Model file for the job. Use its own axes, mm. A direction names the side the tool comes from. Give positions to 0.01 mm unless a question says otherwise; leave off trailing zeros. Order: outer loops, then holes, each group sorted by start corner. A loop starts at its lowest first (then second) coordinate and runs counter-clockwise, first axis right, second up. Notation, with made-up numbers: M 65,76.25 L 113,76.25 A21 cw 113,103.25 Z; hole C 71,-5 d9. An arc over 180 degrees is marked long. Return JSON: item names as keys, results as strings. Group by question number.
1. Wall check: probe 1 along X at (y, z) = (0, -3.5); probe 2 along X at (y, z) = (1, -6). Give the ranges that are in metal, low to high. Write a range as [from, to].
2. Two-plate mould, pull along X, no slides. Class faces 4 (the face through (0, 1, 1)), 5 (the face through (2.11, -5.85, 1.34)), 6 (the face through (1, 0, 1)): released by +X, released by -X, zero draft, split by the parting line, or undercut.
3. 3-axis set-ups, long thin cutter, end or side, ignore diameter. For faces 1 (the face through (1.34, 2.11, -5.85)), 2 (the face through (1, 1, 0)), 3 (the face through (-5.85, 1.69, 1.84)): which of +Z, -Z, +X, -X, +Y, -Y reach the whole face in a straight line?
4. Slice it at D-D on x = -6.75. List the corners of the cut face in (y, z), then the cut area to 3 significant figures.
5. Pin check, flat tips, straight feed: pin 1 (10 mm diameter, centred on x = 5, y = -5.5, fed in from +Z); pin 2 (4.5 mm diameter, centred on x = 0, z = 0, fed in from -Y); pin 3 (4 mm diameter, centred on x = 0, y = 0, fed in from -Z). Stop position of each tip, or through.
6. Slice it at B-B on y = 8. List the corners of the cut face in (x, z), then the cut area to 3 significant figures.
7. Slice it at A-A on z = -8. List the corners of the cut face in (x, y), then the cut area to 3 significant figures.
from build123d import *

# Parameters (mm, degrees)
SKETCH_2_R          = 2.5
CUT_EXTRUDE_1_DEPTH = 18.320508076
SKETCH_3_R          = 2.5
CUT_EXTRUDE_2_DEPTH = 18.320508076
SKETCH_4_R          = 2.5
CUT_EXTRUDE_3_DEPTH = 18.320508076


with BuildPart() as part:
    # 草图1 → 旋转1 (revolve)
    with BuildSketch(Plane(origin=(0, 0, 0), x_dir=(1, 0, 0), z_dir=(0, 1, 0))):
        with BuildLine():
            Line((0, 10), (0, -10))
            ThreePointArc((0, -10), (10, 0), (0, 10))
        make_face()
    revolve(axis=Axis((0, 0, -16.747658197), (0, 0, 1)))

    # 草图2 → 切除-拉伸1 (cut, through all)
    with BuildSketch(Plane(origin=(0, 0, 0), x_dir=(1, 0, 0), z_dir=(0, 1, 0))):
        with Locations(Location((0, 0, 0), (0, 0, 270))):
            Circle(SKETCH_2_R)
    extrude(amount=-CUT_EXTRUDE_1_DEPTH, mode=Mode.SUBTRACT)

    # 草图3 → 切除-拉伸2 (cut, through all)
    with BuildSketch(Plane(origin=(0, 0, 0), x_dir=(0, 0, -1), z_dir=(1, 0, 0))):
        Circle(SKETCH_3_R)
    extrude(amount=-CUT_EXTRUDE_2_DEPTH, mode=Mode.SUBTRACT)

    # 草图4 → 切除-拉伸3 (cut, through all)
    with BuildSketch(Plane.XY):
        Circle(SKETCH_4_R)
    extrude(amount=-CUT_EXTRUDE_3_DEPTH, mode=Mode.SUBTRACT)


solid = part.part
Result:
{
 "1": {"probe 1": "x = [-9.37, -2.5], [2.5, 9.37]", "probe 2": "x = [-7.94, -2.29], [2.29, 7.94]"},
 "2": {"face 4": "released by -X", "face 5": "undercut", "face 6": "zero draft"},
 "3": {"face 1": "-Z", "face 2": "-Z, -X, -Y", "face 3": "-X"},
 "4": {"outline": "C 0,0 d14.76; hole C 0,0 d5", "area": "151 mm2"},
 "5": {"pin 1": "stops at z = 9.7", "pin 2": "stops at y = 0", "pin 3": "stops at z = 0"},
 "6": {"outline": "C 0,0 d12", "area": "113 mm2"},
 "7": {"outline": "C 0,0 d12; hole C 0,0 d5", "area": "93.5 mm2"}
}
